Design review of the part built by this model. Coordinates are the model's own, in mm. Face numbers are marked on the shaded views. A direction names the side the tool comes from. Coordinates: 2 decimals unless noted, no trailing zeros. Loops run counter-clockwise (first coordinate to the right, second up) from the corner with the lowest first, then second, coordinate; pieces in that order, holes last. Notation, with made-up numbers: (38.25, 28.25) - (84.25, 28.25) arc R27 cw to (84.25, 66.25) - close; hole circle Ø11 at (38.25, 75). An arc over 180 degrees is marked (long way). Use one line per item in the form item = value. Start each with the question number.
(1) Tool access review of the marked faces 4 and 5: name each direction out of +Z, -Z, +X, -X, +Y, -Y from which nothing blocks a thin tool from reaching the whole face with its end or side.
(2) Clearance check with flat-ended pins moving along their axes: pin 1 Ø1.5 at (y, z) = (-2.5, -1.5) entering from +X; pin 2 Ø1 at (x, y) = (1.5, -1.5) entering from -Z; pin 3 Ø1.5 at (x, y) = (-1, 1.5) entering from +Z. State where each tip first meets the part, or that it passes through.
(3) Add section C-C (x = 0.75). State the section outline as (y, z) points.
(4) Add section B-B (z = 0). State the section outline as (x, y) points.
(5) The part is to be moulded in two halves that separate along Z. For the marked faces 1, 2 and 3, say which applies: pulls with the +Z half, pulls with the -Z half, needs draft (parallel to the pull), parting line crosses it, or undercut.
(6) Add section A-A (y = 7). State the section outline as (x, z) points (3 decimals), plus the area to 3 significant figures.
(7) For L1, parallel to X at y = 6.25, z = 0; L2, parallel to Z at x = 1, y = 7; L3, parallel to Y at x = 1.85, z = 0.75, list the stretches that pass through material, from the lowest coordinate up.
(8) Add section D-D (y = 4). State the section outline as (x, z) points (3 decimals), plus the area to 3 significant figures.
```python
from build123d import *

# Parameters (mm, degrees)
EXTRUDE_1_DEPTH     = 8
SKETCH_2_R          = 1.5
CUT_EXTRUDE_1_DEPTH = 3
SKETCH_3_R          = 1.5
EXTRUDE_2_DEPTH     = 5


with BuildPart() as part:
    # 草图1 → 凸台-拉伸1 (new body)
    with BuildSketch(Plane(origin=(0, 0, 0), x_dir=(1, 0, 0), z_dir=(0, 1, 0))):
        Polygon((0, 2.35), (-2.035159699, 1.175), (-2.035159699, -1.175), (0, -2.35), (2.035159699, -1.175), (2.035159699, 1.175), align=None)
    extrude(amount=EXTRUDE_1_DEPTH)

    # 草图2 → 切除-拉伸1 (cut)
    with BuildSketch(Plane(origin=(0, 8, 0), x_dir=(1, 0, 0), z_dir=(0, 1, 0))):
        with Locations(Location((0, 0, 0), (0, 0, 270))):
            Circle(SKETCH_2_R)
    extrude(amount=-CUT_EXTRUDE_1_DEPTH, mode=Mode.SUBTRACT)

    # 草图3 → 凸台-拉伸2 (add)
    with BuildSketch(Plane.XZ):
        with Locations(Location((0, 0, 0), (0, 0, 90))):
            Circle(SKETCH_3_R)
    extrude(amount=EXTRUDE_2_DEPTH)


solid = part.part
```
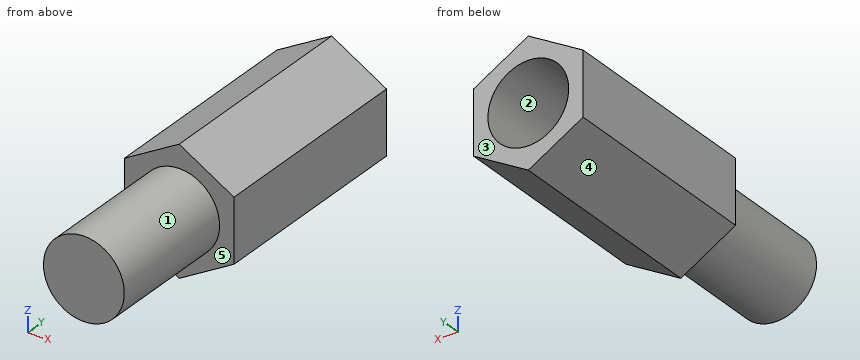
Computed values:
q1.face_4 = -Z, -X, +Y, -Y
q1.face_5 = -Y
q2.pin_1 = 1.3
q2.pin_2 = -1.12
q2.pin_3 = 2.21
q3.outline = (-5, -1.3) - (0, -1.3) - (0, -1.92) - (8, -1.92) - (8, -1.3) - (5, -1.3) - (5, 1.3) - (8, 1.3) - (8, 1.92) - (0, 1.92) - (0, 1.3) - (-5, 1.3) - close
q4.outline = (-2.04, 0) - (-1.5, 0) - (-1.5, -5) - (1.5, -5) - (1.5, 0) - (2.04, 0) - (2.04, 8) - (1.5, 8) - (1.5, 5) - (-1.5, 5) - (-1.5, 8) - (-2.04, 8) - close
q5.face_1 = parting line crosses it
q5.face_2 = undercut
q5.face_3 = needs draft
q6.outline = (-2.035, -1.175) - (0, -2.35) - (2.035, -1.175) - (2.035, 1.175) - (0, 2.35) - (-2.035, 1.175) - close; hole circle Ø3 at (0, 0)
q6.area = 7.28 mm^2
q7.L1 = -2.04 to -1.5, 1.5 to 2.04
q7.L2 = -1.77 to -1.12, 1.12 to 1.77
q7.L3 = 0 to 8
q8.outline = (-2.035, -1.175) - (0, -2.35) - (2.035, -1.175) - (2.035, 1.175) - (0, 2.35) - (-2.035, 1.175) - close
q8.area = 14.3 mm^2
